```python
from build123d import *

# Parameters (mm, degrees)
SKETCH1_W           = 40.5
SKETCH1_H           = 40.5
BOSS_EXTRUDE1_DEPTH = 3
SKETCH1_3_W         = 40.5
SKETCH1_3_H         = 40.5
SKETCH1_3_W_2       = 3
SKETCH1_3_H_2       = 16
BOSS_EXTRUDE2_DEPTH = 1


with BuildPart() as part:
    # Sketch1 → Boss-Extrude1 (new body)
    with BuildSketch(Plane(origin=(0, 0, 0), x_dir=(1, 0, 0), z_dir=(0, 1, 0))):
        with BuildLine():
            Line((-19.9, 37.4), (19.9, 37.4))
            ThreePointArc((19.9, 37.4), (21.667766953, 36.667766953), (22.4, 34.9))
            Line((22.4, 34.9), (22.4, -34.9))
            ThreePointArc((22.4, -34.9), (21.667766953, -36.667766953), (19.9, -37.4))
            Line((19.9, -37.4), (-19.9, -37.4))
            ThreePointArc((-19.9, -37.4), (-21.667766953, -36.667766953), (-22.4, -34.9))
            Line((-22.4, -34.9), (-22.4, 34.9))
            ThreePointArc((-22.4, 34.9), (-21.667766953, 36.667766953), (-19.9, 37.4))
        make_face()
        with Locations((0, -15.15)):
            Rectangle(SKETCH1_W, SKETCH1_H, mode=Mode.SUBTRACT)
    extrude(amount=BOSS_EXTRUDE1_DEPTH)

    # Sketch1_3 → Boss-Extrude2 (add)
    with BuildSketch(Plane(origin=(0, 0, 0), x_dir=(1, 0, 0), z_dir=(0, 1, 0))):
        with Locations((0, -15.15)):
            Rectangle(SKETCH1_3_W, SKETCH1_3_H)
        with Locations((-17.25, -24.9)):
            Rectangle(SKETCH1_3_W_2, SKETCH1_3_H_2, mode=Mode.SUBTRACT)
    extrude(amount=BOSS_EXTRUDE2_DEPTH)


solid = part.part
```
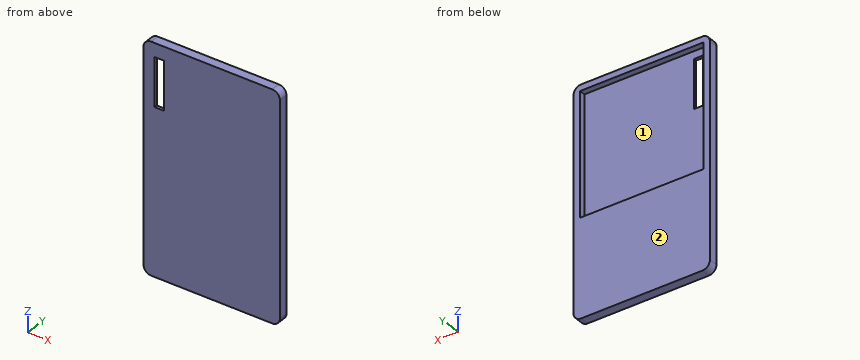
Input: part model. Units: mm. Frame: model coordinates. Face numbers are marked on the shaded views. A direction names the side the tool comes from. Round coordinates to 2 decimals unless told otherwise and drop trailing zeros. Order: outer loops, then holes, each group sorted by start corner. A loop starts at its lowest first (then second) coordinate and runs counter-clockwise, first axis right, second up. Notation, with made-up numbers: (-37, 11) - (-24, 11) arc R10 cw to (-24, 28) - close; hole circle Ø11 at (-38, -29). An arc over 180 degrees is marked (long way). Answer in a Markdown table with one row per item.
Item 1: Reachability of the marked faces 1 and 2 from +Z, -Z, +X, -X, +Y, -Y: full face, straight path, thin tool, end or side. Return the list, or none.
Model answer:
| item | result |
|---|---|
| face 1 | +Y |
| face 2 | +Z, -Z, +X, -X, +Y |
Item 2: Line query: line 1 (Z direction, x = -3.5, y = 2.4); line 2 (X direction, y = 1.8, z = -1); line 3 (X direction, y = 0.85, z = 27.5). Output: solid intervals per line, ascending.
Model answer:
| item | result |
|---|---|
| line 1 | z = -37.4 to -5.1, 35.4 to 37.4 |
| line 2 | x = -22.4 to -20.25, 20.25 to 22.4 |
| line 3 | x = -22.4 to -18.75, -15.75 to 22.4 |
Item 3: Section query B-B (z = 21.5). Return the cut outline in (x, y).
Model answer:
| item | result |
|---|---|
| outline | (-22.4, 0) - (-18.75, 0) - (-18.75, 1) - (-20.25, 1) - (-20.25, 3) - (-22.4, 3) - close; (-15.75, 0) - (22.4, 0) - (22.4, 3) - (20.25, 3) - (20.25, 1) - (-15.75, 1) - close |
Item 4: Section query C-C (y = 2.3). Return the cut outline in (x, z).
Model answer:
| item | result |
|---|---|
| outline | (-22.4, -34.9) arc R2.5 ccw to (-19.9, -37.4) - (19.9, -37.4) arc R2.5 ccw to (22.4, -34.9) - (22.4, 34.9) arc R2.5 ccw to (19.9, 37.4) - (-19.9, 37.4) arc R2.5 ccw to (-22.4, 34.9) - close; hole (-20.25, -5.1) - (20.25, -5.1) - (20.25, 35.4) - (-20.25, 35.4) - close |
Item 5: Pin query (flat end, axial travel): pin 1 (2 mm diameter, centred on x = -9.5, z = -2.5, fed in from +Y). Return the tip coordinate at first contact, or that it passes through.
Model answer:
| item | result |
|---|---|
| pin 1 | stops at y = 1 |
Item 6: Section query D-D (z = 5). Return the cut outline in (x, y).
Model answer:
| item | result |
|---|---|
| outline | (-22.4, 0) - (22.4, 0) - (22.4, 3) - (20.25, 3) - (20.25, 1) - (-20.25, 1) - (-20.25, 3) - (-22.4, 3) - close |
Item 7: Section query A-A (x = 18.5). Return the cut outline in (y, z), then the cut area to 3 significant figures.
Model answer:
| item | result |
|---|---|
| outline | (0, -37.4) - (3, -37.4) - (3, -5.1) - (1, -5.1) - (1, 35.4) - (3, 35.4) - (3, 37.4) - (0, 37.4) - close |
| area | 143 mm² |
